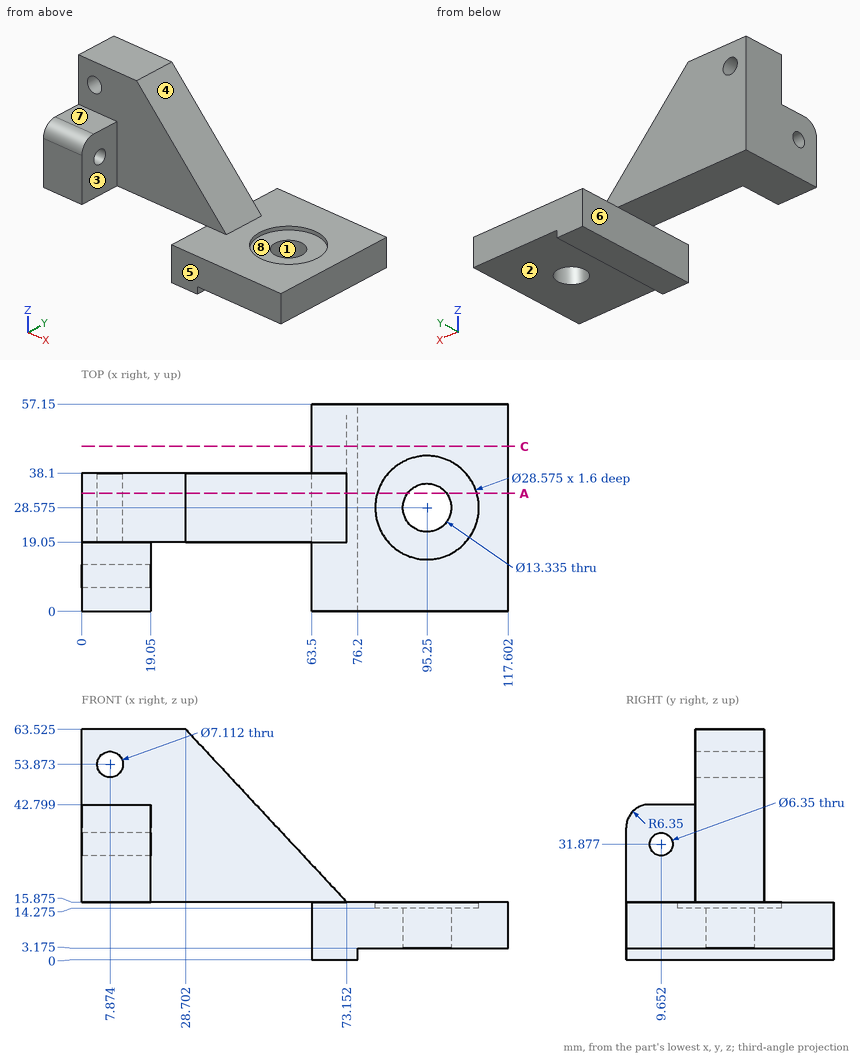
Print and shaded views of the part. All mm, measured from the part's lowest x, y and z. A direction names the side the tool comes from. Coordinates: 2 decimals unless noted, no trailing zeros. Loops run counter-clockwise (first coordinate to the right, second up) from the corner with the lowest first, then second, coordinate; pieces in that order, holes last. Notation, with made-up numbers: M 79,63 L 134,63 A22 ccw 134,78 Z; hole C -27,0.5 d6. An arc over 180 degrees is marked long. Use a Markdown table: item, result. Add a question column.
Q1. Which spindle directions (+Z, -Z, +X, -X, +Y, -Y) get a long thin tool onto all of the face, cutting with end or side? Do the marked faces 4, 5, 6, 7 and 8. Say none if no direction does.
Q2. Mould opens along X. For the marked faces 1, 2 and 3 say: +X half, -X half, draft (parallel to the pull), parting line (faces both ways), or undercut.
Q3. Cut at C-C (y = 45.5). Write the cut outline in (x, z) (1 decimal).
Q4. Probe L1, parallel to Y at x = 95, z = 15; L2, parallel to Y at x = 37, z = 26; L3, parallel to Z at x = 108.5, y = 54 (1 decimal). List the from-to ranges inside material, lowest first.
Q5. Cut at A-A (y = 32.5). Write the cut outline in (x, z) (1 decimal), and give its area (3 significant figures).
Q6. Pin check, flat tips, straight feed: P1, Ø15, axis at y = 6.5, z = 27, coming from the +X side; P2, Ø23, axis at x = 91, y = 30.5, coming from the +Z side (3 decimals); P3, Ø4, axis at y = 6.5, z = 8.5, coming from the -X side. Stop position of each tip, or through.
Worked out:
| question | item | result |
|---|---|---|
| 1 | face 4 | +Z, +X, +Y, -Y |
| 1 | face 5 | +Z, -Z, +X, -X, -Y |
| 1 | face 6 | -Z, -X, +Y, -Y |
| 1 | face 7 | +Z, +X, -X, -Y |
| 1 | face 8 | +Z |
| 2 | face 1 | undercut |
| 2 | face 2 | draft |
| 2 | face 3 | +X half |
| 3 | outline | M 63.5,0 L 76.2,0 L 76.2,3.2 L 117.6,3.2 L 117.6,15.9 L 63.5,15.9 Z |
| 4 | L1 | y = 0 to 14.29, 42.86 to 57.15 |
| 4 | L2 | y = 19.05 to 38.1 |
| 4 | L3 | z = 3.2 to 15.9 |
| 5 | outline | M 0,15.9 L 63.5,15.9 L 63.5,0 L 76.2,0 L 76.2,3.2 L 89.9,3.2 L 89.9,14.3 L 81.5,14.3 L 81.5,15.9 L 73.2,15.9 L 28.7,63.5 L 0,63.5 Z; M 100.6,3.2 L 117.6,3.2 L 117.6,15.9 L 109,15.9 L 109,14.3 L 100.6,14.3 Z; hole C 7.9,53.9 d7.1 |
| 5 | area | 2,950 mm2 |
| 6 | P1 | stops at x = 19.05 |
| 6 | P2 | stops at z = 15.875 |
| 6 | P3 | stops at x = 63.5 |
